from build123d import *

# Parameters (mm, degrees)
IZIM1_R                     = 2.75
Y_KSEKLIK_EKSTR_ZYON1_DEPTH = 40
IZIM2_R                     = 2.75
IZIM2_W                     = 7.285533906
IZIM2_H                     = 10
KES_EKSTR_ZYON1_DEPTH       = 40
PAH1_SIZE                   = 2.5


with BuildPart() as part:
    # Çizim1 → Yükseklik-Ekstrüzyon1 (new body)
    with BuildSketch(Plane.XY):
        with BuildLine():
            Line((-4.545775403, 5), (11.152492002, 5))
            Line((11.152492002, 5), (11.152492002, 0))
            Line((11.152492002, 0), (-8.847507998, 0))
            ThreePointArc((-8.847507998, 0), (-11.909370176, 5.915063509), (-5.311974092, 5))
            Line((-5.311974092, 5), (-4.545775403, 5))
        make_face()
        with Locations((-8.847507998, 3.75)):
            Circle(IZIM1_R, mode=Mode.SUBTRACT)
    extrude(amount=Y_KSEKLIK_EKSTR_ZYON1_DEPTH)

    # Çizim2 → Kes-Ekstrüzyon1 (cut)
    with BuildSketch(Plane(origin=(0, 0, 0), x_dir=(1, 0, 0), z_dir=(0, 1, 0))):
        with Locations(Location((1.152492002, -7.5, 0), (0, 0, 90))):
            Circle(IZIM2_R)
        with Locations(Location((1.152492002, -32.5, 0), (0, 0, 90))):
            Circle(IZIM2_R)
        with Locations((-8.954741045, -35)):
            Rectangle(IZIM2_W, IZIM2_H)
        with Locations((-8.954741045, -15)):
            Rectangle(IZIM2_W, IZIM2_H)
    extrude(amount=KES_EKSTR_ZYON1_DEPTH, mode=Mode.SUBTRACT)

    # Pah1
    pah1_edges = [part.edges().sort_by_distance(p)[0] for p in [
        (2.920258955, 5, 40),
        (2.920258955, 5, 0),
        (11.152492002, 5, 20),
    ]]
    chamfer(pah1_edges, length=PAH1_SIZE)


solid = part.part
CAD build for the part. Positions are in the model's coordinates, mm. A direction names the side the tool comes from. Round coordinates to 2 decimals unless told otherwise and drop trailing zeros. Write each loop counter-clockwise with the first axis right and the second up, starting at its lowest first coordinate (ties: lowest second). Pieces come first, ordered by that corner, then holes. Notation, with made-up numbers: (1.25, 87) -> (38.25, 87) arc R14 cw to (38.25, 109) -> close; hole circle Ø3 at (-40, -12). An arc over 180 degrees is marked (long way). Answer as a JSON object with one key per item and string values.
(1) Band-saw the part on C-C, the plane y = 3.75. List the corners of the cut face in (x, z), then the cut area to 3 significant figures.
Reported:
{"outline": "(-12.6, 0) -> (-11.6, 0) -> (-11.6, 10) -> (-12.6, 10) -> close; (-12.6, 20) -> (-11.6, 20) -> (-11.6, 30) -> (-12.6, 30) -> close; (-6.1, 0) -> (-5.1, 0) -> (-5.1, 1.25) -> (9.9, 1.25) -> (9.9, 38.75) -> (-5.31, 38.75) -> (-5.31, 30) -> (-6.1, 30) -> (-6.1, 20) -> (-5.31, 20) -> (-5.31, 10) -> (-6.1, 10) -> close; hole circle Ø5.5 at (1.15, 7.5); hole circle Ø5.5 at (1.15, 32.5)", "area": "559 mm^2"}
(2) Band-saw the part on D-D, the plane x = 0.75. List the corners of the cut face in (y, z), then the cut area to 3 significant figures.
Reported:
{"outline": "(0, 0) -> (2.5, 0) -> (5, 2.5) -> (5, 4.78) -> (0, 4.78) -> close; (0, 10.22) -> (5, 10.22) -> (5, 29.78) -> (0, 29.78) -> close; (0, 35.22) -> (5, 35.22) -> (5, 37.5) -> (2.5, 40) -> (0, 40) -> close", "area": "139 mm^2"}
(3) Pin check, flat tips, straight feed: P1, Ø8, axis at x = 3.5, z = 10, coming from the +Y side; P2, Ø4.5, axis at x = 1.15, z = 32.5, coming from the +Y side; P3, Ø2, axis at x = -5.5, z = 30, coming from the +Y side. Stop position of each tip, or through.
Reported:
{"P1": "stops at y = 5", "P2": "passes through", "P3": "stops at y = 6.67"}
(4) Probe probe 1 along X at (y, z) = (2.25, 7.5); probe 2 along Z at (x, y) = (2.5, 2.75); probe 3 along Y at (x, z) = (4.25, 24). List the from-to ranges inside material, lowest first. Write a range as [from, to].
Reported:
{"probe 1": "x = [-12.28, -11.15], [-6.54, -1.6], [3.9, 11.15]", "probe 2": "z = [0.25, 5.1], [9.9, 30.1], [34.9, 39.75]", "probe 3": "y = [0, 5]"}
(5) Which spindle directions (+Z, -Z, +X, -X, +Y, -Y) get a long thin tool onto all of the face, cutting with end or side? Do faces 4 (the face through (-5.312, 2, 35)), 5 (the face through (-7, 1, 20)), 6 (the face through (2, 5, 20)), 7 (the face through (4, 0, 20)). Say none if no direction does.
Reported:
{"face 4": "+Z, -X, +Y, -Y", "face 5": "-X, +Y, -Y", "face 6": "+Z, -Z, +X, +Y", "face 7": "+Z, -Z, +X, -X, -Y"}
(6) Band-saw the part on B-B, the plane z = 32.5. List the corners of the cut face in (x, y), then the cut area to 3 significant figures.
Reported:
{"outline": "(-5.31, 0) -> (-1.6, 0) -> (-1.6, 5) -> (-5.31, 5) -> close; (3.9, 0) -> (11.15, 0) -> (11.15, 2.5) -> (8.65, 5) -> (3.9, 5) -> close", "area": "51.7 mm^2"}
(7) Band-saw the part on A-A, the plane z = 7.5. List the corners of the cut face in (x, y).
Reported:
{"outline": "(-8.85, 0) -> (-1.6, 0) -> (-1.6, 5) -> (-5.31, 5) arc R3.75 ccw (long way) to start; (3.9, 0) -> (11.15, 0) -> (11.15, 2.5) -> (8.65, 5) -> (3.9, 5) -> close; hole circle Ø5.5 at (-8.85, 3.75)"}
(8) Two-plate mould, pull along X, no slides. Class faces 1 (the face through (-9.444, 1.065, 4.93)), 2 (the face through (9.88, 3.77, 19.72)), 3 (the face through (3, 1, 40)): +X half, -X half, draft (parallel to the pull), parting line (faces both ways), or undercut.
Reported:
{"face 1": "undercut", "face 2": "+X half", "face 3": "draft"}
